For this review, take the finished solid that the model builds, in its own axes (mm). A direction names the side the tool comes from. Coordinates: 2 decimals unless noted, no trailing zeros. Order: outer loops, then holes, each group sorted by start corner. A loop starts at its lowest first (then second) coordinate and runs counter-clockwise, first axis right, second up. Notation, with made-up numbers: (89, 33.5) -> (105, 33.5) arc R16 cw to (105, 60.5) -> close; hole circle Ø6 at (-2.75, -1). An arc over 180 degrees is marked (long way). Write item = value, one per line. Start each with the question number.
1) Consider section B-B on z = 14.5. Give the boundary of the cut face in (x, y).
2) Consider section A-A on x = -31. Give the boundary of the cut face in (y, z).
3) Consider section D-D on z = 45. Give the boundary of the cut face in (x, y).
4) Draft analysis for pull direction Y (two halves, no side actions). For faces 4 (the face through (2, -39, 13)), 5 (the face through (29, 77.5, 4)), 6 (the face through (-2, -39, 13)), 7 (the face through (32.18, 76.02, 2.21)), state which applies: +Y half, -Y half, draft (parallel to the pull), parting line (faces both ways), or undercut.
5) Wall thickness on probe 1 along X at (y, z) = (76.85, 3.5); probe 2 along Z at (x, y) = (1.5, 22); probe 3 along Y at (x, z) = (-4, 36): over which ranges is each line inside the solid? List them lowest first. Write a range as [from, to].
6) Insertion check: pin 1 Ø8 at (x, z) = (-32, 2.5) entering from +Y; pin 2 Ø2 at (y, z) = (-43, 21.5) entering from +X; pin 3 Ø10 at (x, y) = (0.5, -38.5) entering from +Z. Each pin has a flat end and moves straight along its axis. Give the tip position at first contact, or say it passes through.
7) Machinability: for faces 1 (the face through (0, 77.5, 4)), 2 (the face through (0, 77, 10.5)), 3 (the face through (-2.4, 1.5, 4)), which of the approach directions +Z, -Z, +X, -X, +Y, -Y give a long, thin tool a straight path to every point of the face, cutting with its end or side? Answer none if there is none.
8) Consider section C-C on y = -38. Give the boundary of the cut face in (x, z).
from build123d import *

# Parameters (mm, degrees)
SKETCH1_W           = 20
SKETCH1_H           = 155
BOSS_EXTRUDE1_DEPTH = 4
SKETCH2_W           = 20
SKETCH2_H           = 4
BOSS_EXTRUDE3_DEPTH = 50
RIB2_REACH          = 96.986
SKETCH7_WALL_W      = 290.205463948
SKETCH7_WALL_H      = 4
SKETCH8_W           = 20
SKETCH8_H           = 3
BOSS_EXTRUDE4_DEPTH = 3.5
SKETCH9_W           = 70
SKETCH9_H           = 5
BOSS_EXTRUDE6_DEPTH = 3
SKETCH10_W          = 10
SKETCH10_H          = 3
BOSS_EXTRUDE7_DEPTH = 7.5
SKETCH12_R          = 1.75
CUT_EXTRUDE1_DEPTH  = 10


with BuildPart() as part:
    # Sketch1 → Boss-Extrude1 (new body)
    with BuildSketch(Plane.XY):
        Rectangle(SKETCH1_W, SKETCH1_H)
    extrude(amount=BOSS_EXTRUDE1_DEPTH)

    # Sketch2 → Boss-Extrude3 (add)
    with BuildSketch(Plane.XY.offset(4)):
        with Locations((0, -75.5)):
            Rectangle(SKETCH2_W, SKETCH2_H)
    extrude(amount=BOSS_EXTRUDE3_DEPTH)

    # Sketch7 wall → Rib2 (add, up to next)
    with BuildSketch(Plane(origin=(0, -26, 16.5), x_dir=(0, 0.967074537263, -0.25449329928), z_dir=(0, 0.25449329928, 0.967074537263)), mode=Mode.PRIVATE) as rib2_sk1:
        Rectangle(SKETCH7_WALL_W, SKETCH7_WALL_H)
    rib2_tool1 = extrude(rib2_sk1.sketch, amount=-RIB2_REACH, mode=Mode.PRIVATE) - part.part
    add(rib2_tool1.solids().sort_by_distance((0, -26, 16.5))[0])

    # Sketch8 → Boss-Extrude4 (add)
    with BuildSketch(Plane.XY.offset(4)):
        with Locations((0, 76)):
            Rectangle(SKETCH8_W, SKETCH8_H)
    extrude(amount=BOSS_EXTRUDE4_DEPTH)

    # Sketch9 → Boss-Extrude6 (add)
    with BuildSketch(Plane.XY.offset(7.5)):
        with Locations((0, 77)):
            Rectangle(SKETCH9_W, SKETCH9_H)
    extrude(amount=BOSS_EXTRUDE6_DEPTH)

    # Sketch10 → Boss-Extrude7 (add)
    with BuildSketch(Plane(origin=(0, 0, 7.5), x_dir=(-1, 0, 0), z_dir=(0, 0, -1))):
        with Locations((30, 76)):
            Rectangle(SKETCH10_W, SKETCH10_H)
        with Locations((-30, 76)):
            Rectangle(SKETCH10_W, SKETCH10_H)
    extrude(amount=BOSS_EXTRUDE7_DEPTH)

    # Sketch12 → Cut-Extrude1 (cut)
    with BuildSketch(Plane(origin=(0, 77.5, 0), x_dir=(1, 0, 0), z_dir=(0, 1, 0))):
        with Locations(Location((-31, -3.5, 0), (0, 0, 270))):
            Circle(SKETCH12_R)
        with Locations(Location((31, -3.5, 0), (0, 0, 270))):
            Circle(SKETCH12_R)
    extrude(amount=-CUT_EXTRUDE1_DEPTH, mode=Mode.SUBTRACT)


solid = part.part
Answer sheet:
q1.outline = (-10, -77.5) -> (10, -77.5) -> (10, -73.5) -> (2, -73.5) -> (2, -18.4) -> (-2, -18.4) -> (-2, -73.5) -> (-10, -73.5) -> close
q2.outline = (74.5, 0) -> (77.5, 0) -> (77.5, 1.75) -> (74.5, 1.75) -> close; (74.5, 5.25) -> (77.5, 5.25) -> (77.5, 7.5) -> (79.5, 7.5) -> (79.5, 10.5) -> (74.5, 10.5) -> close
q3.outline = (-10, -77.5) -> (10, -77.5) -> (10, -73.5) -> (-10, -73.5) -> close
q4.face_4 = undercut
q4.face_5 = +Y half
q4.face_6 = undercut
q4.face_7 = draft
q5.probe_1 = [-35, -32.75], [-29.25, -25], [-10, 10], [25, 29.25], [32.75, 35]
q5.probe_2 = [0, 4]
q5.probe_3 = [-77.5, -73.5]
q6.pin_1 = 77.5
q6.pin_2 = 2
q6.pin_3 = 21.11
q7.face_1 = -Z, +X, -X, +Y
q7.face_2 = +Z, +X, -X, +Y
q7.face_3 = +Z
q8.outline = (-10, 0) -> (10, 0) -> (10, 4) -> (2, 4) -> (2, 19.66) -> (-2, 19.66) -> (-2, 4) -> (-10, 4) -> close
